Can you work these out from the model? Positions are in its coordinate system, mm. A direction names the side the tool comes from. Give positions to 0.01 mm unless a question says otherwise; leave off trailing zeros. Loops run counter-clockwise (first coordinate to the right, second up) from the corner with the lowest first, then second, coordinate; pieces in that order, holes last. Notation, with made-up numbers: (65, 44.5) -> (115, 44.5) arc R15 cw to (115, 48.5) -> close; hole circle Ø6 at (-7.75, -4). An arc over 180 degrees is marked (long way). Use CSV: the item, a comma, the result in double quotes.
Autodesk Inventor part; units mm, degrees
ref_plane "YZ Plane" through (0, 0, 0) normal (1, 0, 0) x (0, 1, 0)
ref_plane "XZ Plane" through (0, 0, 0) normal (0, 1, 0) x (-1, 0, 0)
ref_plane "XY Plane" through (0, 0, 0) normal (0, 0, 1) x (1, 0, 0)
sketch "Boceto1" plane through (0, 0, 0) normal (0, 0, 1) x (1, 0, 0)
  circle A0 centre (0, 0) radius 5
  dimension "d0" = 5
extrude "Extrusión1" add sketch "Boceto1" along normal blind 310
thread "Rosca1"
fillet "Empalme1" radius 2 1 edges at (-5, 0, 310)
sketch "Boceto2" plane through (0, 0, 0) normal (0, 1, 0) x (-1, 0, 0)
  line L0 (-3, 310) -> (3, 310) construction
  line L1 (0, 310) -> (0, 0) construction
  line L2 (-5, 0) -> (-5, 308) construction
  line L3 (5, 0) -> (5, 308)
  line L4 (5, 300) -> (4, 300)
  line L5 (4, 300) -> (4, 301.5)
  line L6 (4, 301.5) -> (5, 301.5)
  line L7 (5, 301.5) -> (5, 300)
  line L8 (5, 0) -> (5, 308)
  line L9 (5, 26.5) -> (4, 26.5)
  line L10 (4, 26.5) -> (4, 25)
  line L11 (4, 25) -> (5, 25)
  line L12 (5, 25) -> (5, 26.5)
  line L13 (-5, 0) -> (5, 0)
  line L14 (5, 272) -> (4, 272)
  line L15 (4, 272) -> (4, 270.5)
  line L16 (4, 270.5) -> (5, 270.5)
  line L17 (5, 270.5) -> (5, 272)
  dimension "d6" = 1.5
  dimension "d7" = 1
  dimension "d9" = 10
  dimension "d11" = 25
  dimension "d12" = 1.5
  dimension "d13" = 1
  dimension "d14" = 1.5
  dimension "d15" = 1
  dimension "d16" = 39.5
revolve "Revolución1" cut sketch "Boceto2" angle 360 about axis through (0, 0, 310) along (0, 0, -1)
properties part number "vailla enroscada" material "Acetal Resin, Black"
(1) If we section it at A-A, the plane z = 143.5: Write out the boundary of the cut face in (x, y), then the cut area to 3 significant figures.
Answer sheet:
outline,"circle Ø10 at (0, 0)"
area,"78.5 mm2"
(2) We'd pull the mould along Z, two halves only. Please class faces 1 (the face through (0, 0, 0)), 2 (the face through (0, 0, 310)), 3 (the face through (-1.08, 4.88, 304.7)), 4 (the face through (0.867, -3.905, 25.74)): released by +Z, released by -Z, zero draft, split by the parting line, or undercut.
Answer sheet:
face 1,"released by -Z"
face 2,"released by +Z"
face 3,"zero draft"
face 4,"undercut"
(3) Which directions (+Z, -Z, +X, -X, +Y, -Y) give clear straight access to the entire face, cutting with the end or side of a thin tool? Please do faces 5 (the face through (-1.08, 4.88, 146.79)), 6 (the face through (0.867, -3.905, 271.24)).
Answer sheet:
face 5,"+Z, -Z"
face 6,"none"
(4) Will these pins go through, and if not, where does the flat tip stop? pin 1 Ø4 at (x, z) = (2, 271) entering from +Y; pin 2 Ø1 at (y, z) = (-3.5, 197) entering from -X.
Answer sheet:
pin 1,"stops at y = 5"
pin 2,"stops at x = -4"
(5) If I drill on L1, parallel to Z at x = 0.75, y = -4.25; L2, parallel to Z at x = 4.5, y = -0.25; L3, parallel to X at y = 0.25, z = 252.5, over which ranges is the centre line in solid material (lowest first)? Write a range as from..to.
Answer sheet:
L1,"z = 0..25, 26.5..270.5, 272..300, 301.5..309.51"
L2,"z = 0..25, 26.5..270.5, 272..300, 301.5..309.31"
L3,"x = -4.99..4.99"
